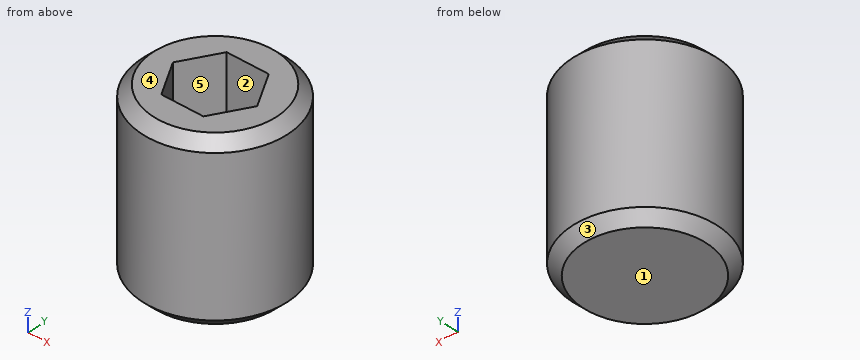
Solid Edge part; units mm, degrees
sketch "Sketch1" plane through (0, 0, 0) normal (0, 0, 1) x (1, 0, 0)
  circle A0 centre (0, 0) radius 7.9375
extrude "Protrusion1" add sketch "Sketch1" along normal blind 19.05
chamfer "Chamfer1" distance 1.1906 angle 45 2 edges at (-7.9375, 0, 0) (-7.9375, 0, 19.05)
sketch "Sketch2" plane through (0, 0, 19.05) normal (0, 0, 1) x (1, 0, 0)
  line L0 (-2.2914, 3.9688) -> (2.2914, 3.9688)
  line L1 (4.5827, 0) -> (2.2914, 3.9687)
  line L2 (2.2914, -3.9688) -> (4.5827, 0)
  line L3 (-2.2914, -3.9688) -> (2.2914, -3.9688)
  line L4 (-4.5827, 0) -> (-2.2914, -3.9688)
  line L5 (-2.2914, 3.9687) -> (-4.5827, 0)
extrude "Cutout1" cut sketch "Sketch2" against normal blind 9.525
properties part number "116405"
Design review of the part built by this model. Coordinates are the model's own, in mm. Face numbers are marked on the shaded views. A direction names the side the tool comes from. Coordinates: 2 decimals unless noted, no trailing zeros. Write each loop counter-clockwise with the first axis right and the second up, starting at its lowest first coordinate (ties: lowest second). Pieces come first, ordered by that corner, then holes.
1) Mouldability with a two-part tool opening along X and no side actions: class the marked faces 1, 2 and 3 as +X half, -X half, draft (parallel to the pull), parting line (faces both ways), or undercut.
2) Insertion check: pin 1 (6 mm diameter, centred on x = 6, z = 6.5, fed in from +Y); pin 2 (5 mm diameter, centred on x = 4.5, z = 5.5, fed in from -Y); pin 3 (2 mm diameter, centred on x = -2.5, z = 6.5, fed in from +Y). Each pin has a flat end and moves straight along its axis. Give the tip position at first contact, or say it passes through.
3) To check wall thickness, follow L1, parallel to Y at x = -1, z = 10.5; L2, parallel to Y at x = 4, z = 12.5; L3, parallel to Z at x = -1.5, y = -0.5 (3 decimals). State the ranges of each line that lie inside material, in increasing order.
4) Machinability: for the marked faces 4 and 5, which of the approach directions +Z, -Z, +X, -X, +Y, -Y give a long, thin tool a straight path to every point of the face, cutting with its end or side? Answer none if there is none.
5) Add section C-C (z = 3). Write out the cut boundary in (x, y) (1 decimal), plus the area to 3 significant figures.
6) Add section A-A (z = 15.5). Write out the cut boundary in (x, y) (1 decimal).
Check result:
1. face 1: draft
1. face 2: undercut
1. face 3: parting line
2. pin 1: stops at y = 7.35
2. pin 2: stops at y = -7.68
2. pin 3: stops at y = 7.79
3. L1: y = -7.87 to -3.97, 3.97 to 7.87
3. L2: y = -6.86 to -1.01, 1.01 to 6.86
3. L3: z = 0 to 9.525
4. face 4: +Z, +X, -X, +Y, -Y
4. face 5: +Z
5. outline: circle Ø15.9 at (0, 0)
5. area: 198 mm2
6. outline: circle Ø15.9 at (0, 0); hole (-4.6, 0) - (-2.3, -4) - (2.3, -4) - (4.6, 0) - (2.3, 4) - (-2.3, 4) - close
